Drawing for the job (mm, zero at the part's lowest x, y, z). Round coordinates to 2 decimals unless told otherwise and drop trailing zeros. Order: outer loops, then holes, each group sorted by start corner. A loop starts at its lowest first (then second) coordinate and runs counter-clockwise, first axis right, second up. Notation, with made-up numbers: (83.5, 12.5) -> (127.5, 12.5) arc R12 ccw to (127.5, 24.5) -> close; hole circle Ø3 at (89, 49). An arc over 180 degrees is marked (long way). Use CSV: the item, a comma, the result in double quotes.
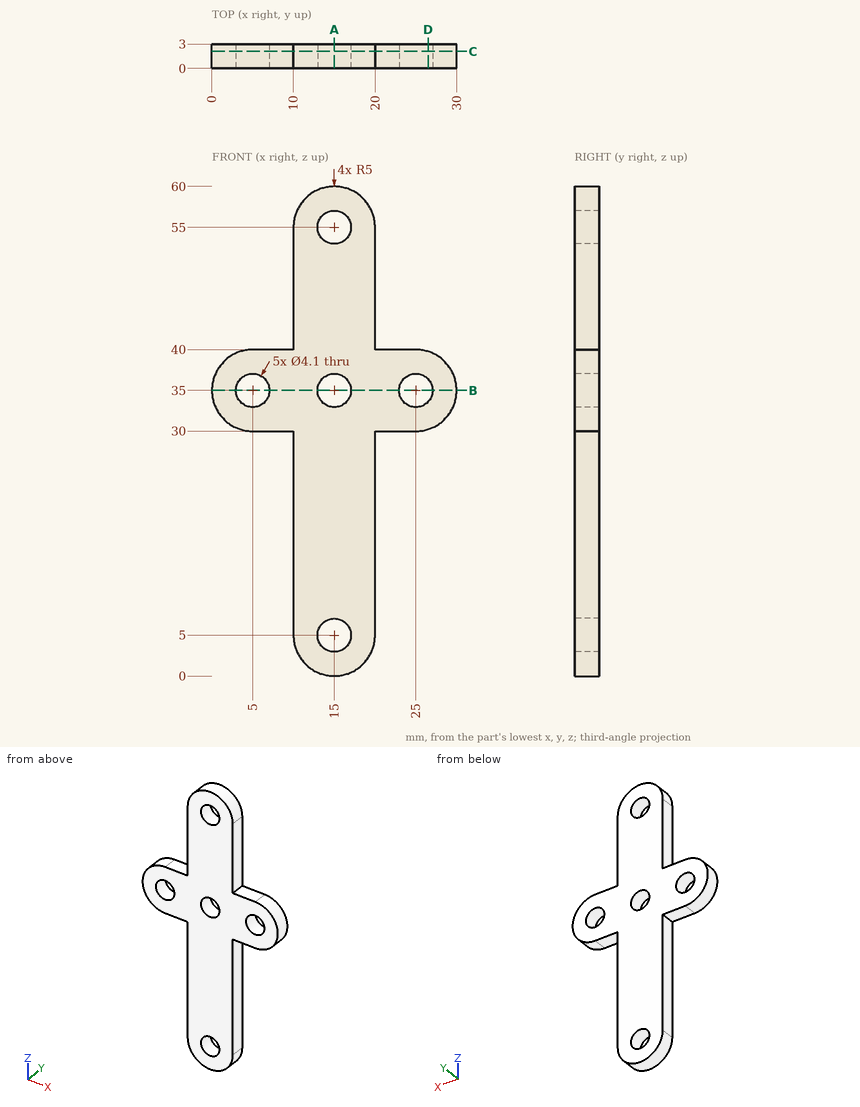
Q1. Cut at D-D (x = 26.5). Give the cut face in (y, z).
From the geometry:
outline,"(0, 30.23) -> (3, 30.23) -> (3, 33.6) -> (0, 33.6) -> close; (0, 36.4) -> (3, 36.4) -> (3, 39.77) -> (0, 39.77) -> close"
Q2. Pin check, flat tips, straight feed: pin 1 (0.9 mm diameter, centred on x = 8.5, y = 1.5, fed in from -Z); pin 2 (1.5 mm diameter, centred on x = 7, y = 2, fed in from +Z); pin 3 (1 mm diameter, centred on y = 1.5, z = 7.5, fed in from -X). Stop position of each tip, or through.
From the geometry:
pin 1,"stops at z = 30"
pin 2,"stops at z = 40"
pin 3,"stops at x = 10"
Q3. Probe line 1 along X through (y, z) = (1.5, 35); line 2 along X through (y, z) = (1.3, 5); line 3 along Z through (x, y) = (5, 0.65). List the from-to ranges inside material, lowest first.
From the geometry:
line 1,"x = 0 to 2.95, 7.05 to 12.95, 17.05 to 22.95, 27.05 to 30"
line 2,"x = 10 to 12.95, 17.05 to 20"
line 3,"z = 30 to 32.95, 37.05 to 40"
Q4. Cut at A-A (x = 15). Give the cut face in (y, z).
From the geometry:
outline,"(0, 0) -> (3, 0) -> (3, 2.95) -> (0, 2.95) -> close; (0, 7.05) -> (3, 7.05) -> (3, 32.95) -> (0, 32.95) -> close; (0, 37.05) -> (3, 37.05) -> (3, 52.95) -> (0, 52.95) -> close; (0, 57.05) -> (3, 57.05) -> (3, 60) -> (0, 60) -> close"
Q5. Cut at B-B (z = 35). Give the cut face in (x, y).
From the geometry:
outline,"(0, 0) -> (2.95, 0) -> (2.95, 3) -> (0, 3) -> close; (7.05, 0) -> (12.95, 0) -> (12.95, 3) -> (7.05, 3) -> close; (17.05, 0) -> (22.95, 0) -> (22.95, 3) -> (17.05, 3) -> close; (27.05, 0) -> (30, 0) -> (30, 3) -> (27.05, 3) -> close"
Q6. Cut at C-C (y = 2.1). Give the cut face in (x, z), plus the area to 3 significant figures.
From the geometry:
outline,"(5, 30) -> (10, 30) -> (10, 5) arc R5 ccw to (20, 5) -> (20, 30) -> (25, 30) arc R5 ccw to (25, 40) -> (20, 40) -> (20, 55) arc R5 ccw to (10, 55) -> (10, 40) -> (5, 40) arc R5 ccw to start; hole circle Ø4.1 at (5, 35); hole circle Ø4.1 at (15, 5); hole circle Ø4.1 at (15, 35); hole circle Ø4.1 at (15, 55); hole circle Ø4.1 at (25, 35)"
area,"691 mm²"
